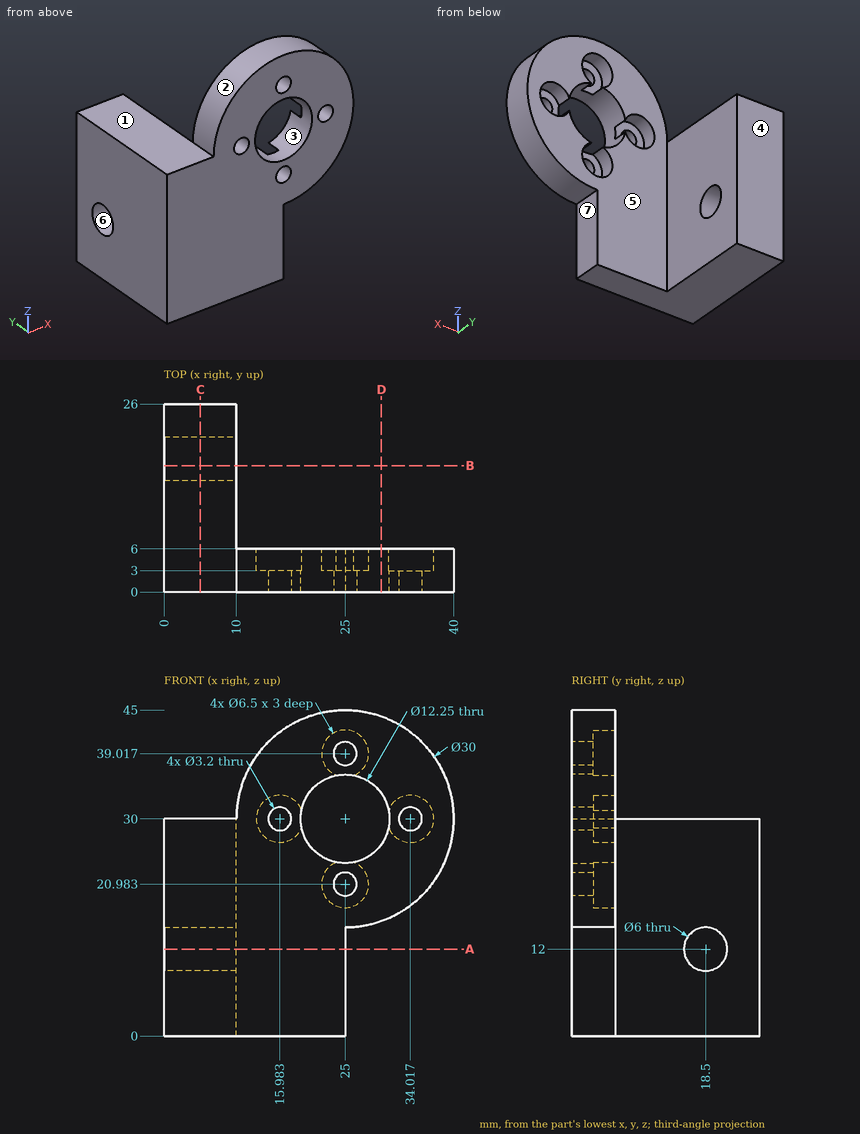
The drawing under review shows one solid part. Ordinate dimensions are in mm from its lowest x, y, z. A direction names the side the tool comes from. Coordinates: 2 decimals unless noted, no trailing zeros. Loops run counter-clockwise (first coordinate to the right, second up) from the corner with the lowest first, then second, coordinate; pieces in that order, holes last. Notation, with made-up numbers: M 37.5,63 L 44.5,63 A10 ccw 44.5,67 Z; hole C 44.25,-38 d9. An arc over 180 degrees is marked long. Use one line per item in the form item = value.
(1) Clearance check with flat-ended pins moving along their axes: P1, Ø5.5, axis at y = 18.5, z = 12, coming from the -X side; P2, Ø3, axis at x = 17, z = 29.5, coming from the +Y side; P3, Ø10, axis at x = 23, z = 32, coming from the +Y side; P4, Ø6, axis at x = 34.017, z = 30, coming from the -Y side. State where each tip first meets the part, or that it passes through.
Return value:
P1 = through
P2 = 3
P3 = 6
P4 = 0
(2) Consider section B-B (y = 17.5). Write out the cut boundary in (x, z).
Return value:
outline = M 0,0 L 10,0 L 10,9.17 L 0,9.17 Z; M 0,14.83 L 10,14.83 L 10,30 L 0,30 Z
(3) Consider section A-A (z = 12). Write out the cut boundary in (x, y), and give its area (3 significant figures).
Return value:
outline = M 0,0 L 25,0 L 25,6 L 10,6 L 10,15.5 L 0,15.5 Z; M 0,21.5 L 10,21.5 L 10,26 L 0,26 Z
area = 290 mm2
(4) Consider section D-D (x = 30). Write out the cut boundary in (y, z), and give its area (3 significant figures).
Return value:
outline = M 0,15.86 L 6,15.86 L 6,26.46 L 0,26.46 Z; M 0,33.54 L 6,33.54 L 6,44.14 L 0,44.14 Z
area = 127 mm2
(5) Consider section C-C (x = 5). Write out the cut boundary in (y, z).
Return value:
outline = M 0,0 L 26,0 L 26,30 L 0,30 Z; hole C 18.5,12 d6
(6) Draft analysis for pull direction Z (two halves, no side actions). For the marked faces 1, 2, 3 and 4, state which applies: pulls with the +Z half, pulls with the -Z half, needs draft (parallel to the pull), parting line crosses it, or undercut.
Return value:
face_1 = pulls with the +Z half
face_2 = parting line crosses it
face_3 = undercut
face_4 = needs draft
(7) For line 1 along Y through (x, z) = (5, 12); line 2 along X through (y, z) = (3.75, 27); line 3 along Y through (x, z) = (33.5, 21), list the stretches that pass through material, from the lowest coordinate up. Write a range as from..to.
Return value:
line_1 = 0..15.5, 21.5..26
line_2 = 0..14.73, 17.23..19.66, 30.34..32.77, 35.27..39.7
line_3 = 0..6
(8) For the marked faces 5, 6 and 7, list the 3-axis set-ups (+Z, -Z, +X, -X, +Y, -Y) from which the entire face can be reached by the end or side of a thin tool; tool diameter is ignored.
Return value:
face_5 = +Z, -Z, +X, +Y
face_6 = +X, -X
face_7 = -Z, +X, +Y, -Y
